Here's the drawing with two shaded views (mm, measured from the low corner). I have some questions. Coordinates: 2 decimals unless noted, no trailing zeros. Loops run counter-clockwise (first coordinate to the right, second up) from the corner with the lowest first, then second, coordinate; pieces in that order, holes last. Notation, with made-up numbers: (75.25, -14.5) -> (99.25, -14.5) arc R20 cw to (99.25, 7.5) -> close; hole circle Ø7 at (87, 19). An arc over 180 degrees is marked (long way). Answer as a JSON object with one key per item and string values. Group by question number.
Q1. I want a section at A-A on y = 29.5. Write out the boundary of the cut face in (x, z).
Q2. I need wall thicknesses on line 1 (Y direction, x = 29.5, z = 1.1); line 2 (Y direction, x = 46.5, z = 0.8) (1 decimal); line 3 (Y direction, x = 12.5, z = 2.2) (1 decimal). Which ranges of each line are inside material? Lowest first, please.
Q3. I'm going to push flat-ended pins straight in: pin 1 (3.5 mm diameter, centred on x = 46.91, y = 29.5, fed in from +Z); pin 2 (1 mm diameter, centred on x = 31, z = 1, fed in from +Y); pin 3 (1 mm diameter, centred on y = 18, z = 0.5, fed in from +X). Where does each tip first touch, or does it pass through?
Q4. I want a section at B-B on x = 29.5. Write out the boundary of the cut face in (y, z), then the cut area to 3 significant figures.
Q5. I want a section at C-C on z = 2.2. Count the separate pieces of the cut face and the enclosed holes in it, then the cut area to 3 significant figures.
Q6. I want a section at D-D on x = 12.25. Write out the boundary of the cut face in (y, z).
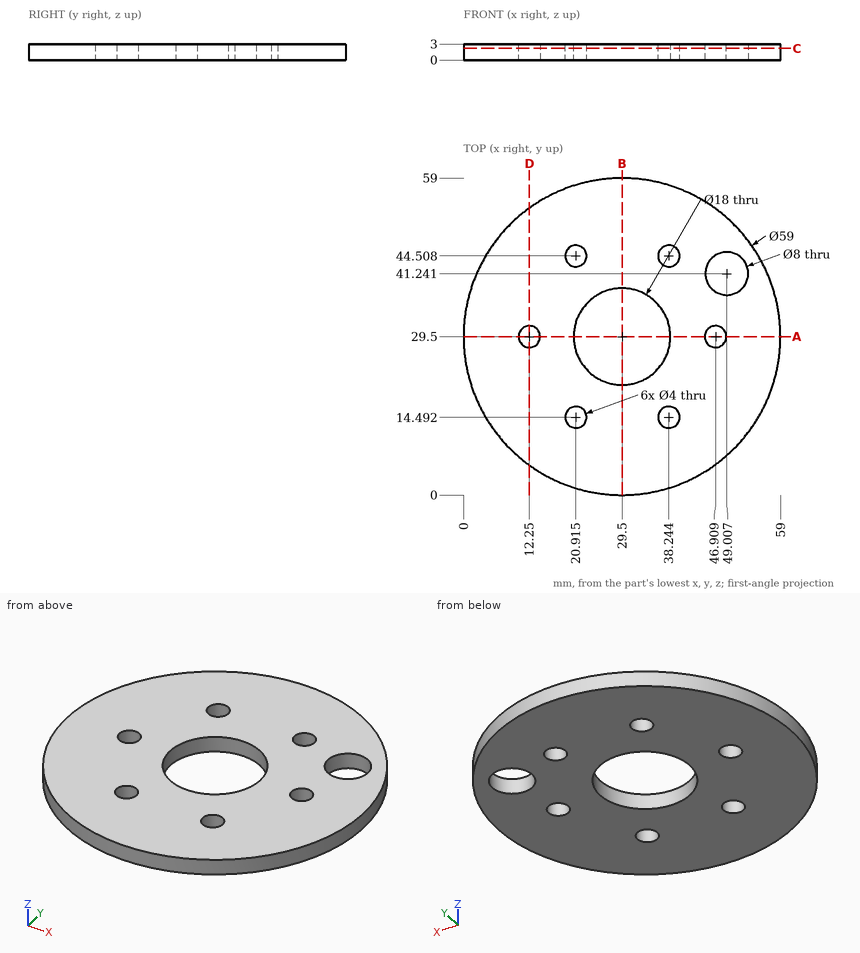
Result set:
{
 "1": {"outline": "(0, 0) -> (10.25, 0) -> (10.25, 3) -> (0, 3) -> close; (14.25, 0) -> (20.5, 0) -> (20.5, 3) -> (14.25, 3) -> close; (38.5, 0) -> (44.91, 0) -> (44.91, 3) -> (38.5, 3) -> close; (48.91, 0) -> (59, 0) -> (59, 3) -> (48.91, 3) -> close"},
 "2": {"line 1": "y = 0 to 20.5, 38.5 to 59", "line 2": "y = 5.4 to 27.5, 31.5 to 38.1, 44.4 to 53.6", "line 3": "y = 5.4 to 27.5, 31.5 to 53.6"},
 "3": {"pin 1": "passes through", "pin 2": "stops at y = 58.98", "pin 3": "stops at x = 56.87"},
 "4": {"outline": "(0, 0) -> (20.5, 0) -> (20.5, 3) -> (0, 3) -> close; (38.5, 0) -> (59, 0) -> (59, 3) -> (38.5, 3) -> close", "area": "123 mm²"},
 "5": {"separate pieces": "1", "enclosed holes": "8", "area": "2,350 mm²"},
 "6": {"outline": "(5.57, 0) -> (27.5, 0) -> (27.5, 3) -> (5.57, 3) -> close; (31.5, 0) -> (53.43, 0) -> (53.43, 3) -> (31.5, 3) -> close"}
}
